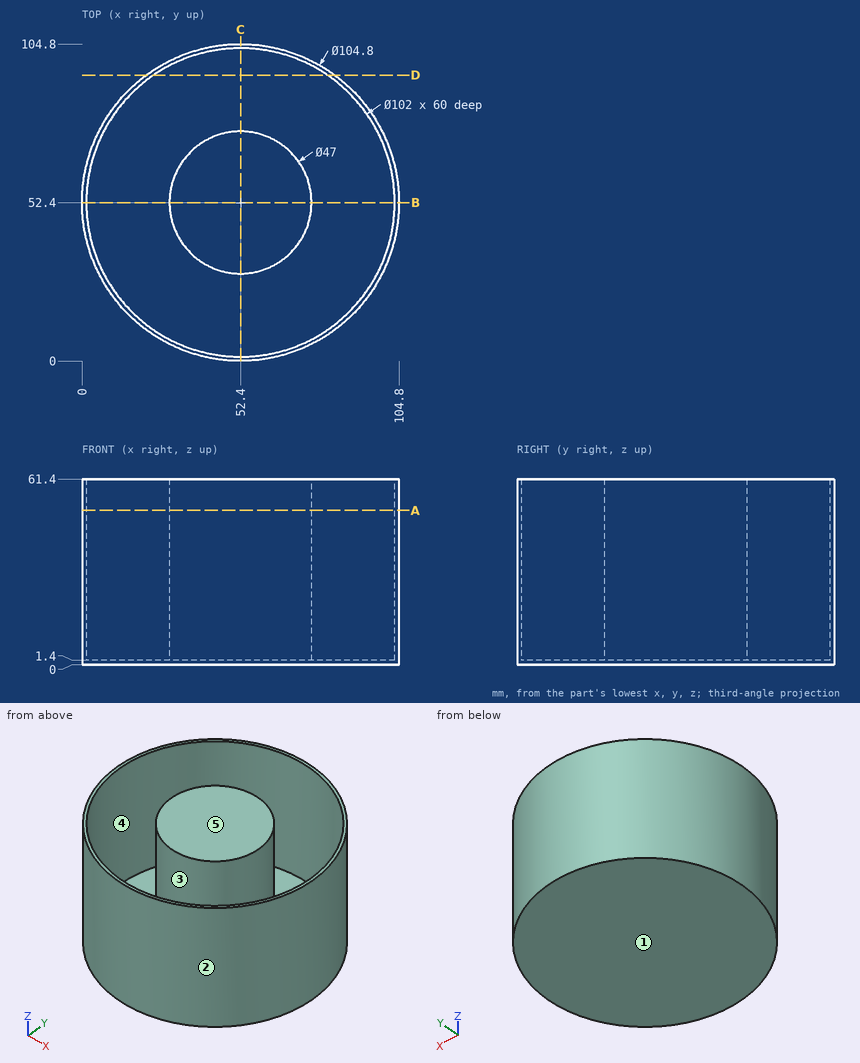
Can you work these out from the drawing? Everything is in mm from the part's minimum corner. A direction names the side the tool comes from. Give positions to 0.01 mm unless a question says otherwise; leave off trailing zeros. Order: outer loops, then holes, each group sorted by start corner. A loop starts at its lowest first (then second) coordinate and runs counter-clockwise, first axis right, second up. Notation, with made-up numbers: M -29.75,-2.5 L 25.25,-2.5 A12 cw 25.25,17.5 Z; hole C 67.5,30.25 d1. An arc over 180 degrees is marked long. One line per item, written item: value.
Item 1: Please list where these lines run through material, in increasing order: line 1 (Y direction, x = 52, z = 40); line 2 (X direction, y = 47.5, z = 53.5).
Verdict:
line 1: 0 to 1.4, 28.9 to 75.9, 103.4 to 104.8
line 2: 0.23 to 1.64, 29.42 to 75.38, 103.16 to 104.57
Item 2: If we section it at A-A on z = 51: Write out the boundary of the cut face in (x, y).
Verdict:
outline: C 52.4,52.4 d104.8; C 52.4,52.4 d47; hole C 52.4,52.4 d102
Item 3: For the marked faces 4 and 5, which set-ups out of +Z, -Z, +X, -X, +Y, -Y let a thin tool reach every point of the face, with its end or its side?
Verdict:
face 4: +Z
face 5: +Z, +X, -X, +Y, -Y
Item 4: If we section it at B-B on y = 52.4: Write out the boundary of the cut face in (x, z), and give its area (3 significant figures).
Verdict:
outline: M 0,0 L 104.8,0 L 104.8,61.4 L 103.4,61.4 L 103.4,1.4 L 75.9,1.4 L 75.9,61.4 L 28.9,61.4 L 28.9,1.4 L 1.4,1.4 L 1.4,61.4 L 0,61.4 Z
area: 3,130 mm2
Item 5: If we mould it in two halves opening along Y, with no side actions, what happens to the marked faces 1, 2 and 3? For each: pulls with the +Y half, pulls with the -Y half, needs draft (parallel to the pull), parting line crosses it, or undercut.
Verdict:
face 1: needs draft
face 2: parting line crosses it
face 3: undercut
Item 6: For pin 1 (2 mm diameter, centred on x = 33, z = 27, fed in from +Y); pin 2 (4 mm diameter, centred on x = 30.5, z = 21.5, fed in from +Y); pin 3 (6 mm diameter, centred on x = 25.5, z = 15.5, fed in from +Y), each with a flat end and sliding along its axis, tell me the tip position at first contact or that it passes through.
Verdict:
pin 1: y = 101.46
pin 2: y = 100.87
pin 3: y = 99.03
Item 7: If we section it at D-D on y = 94.5: Write out the boundary of the cut face in (x, z).
Verdict:
outline: M 21.2,0 L 83.6,0 L 83.6,61.4 L 81.19,61.4 L 81.19,1.4 L 23.61,1.4 L 23.61,61.4 L 21.2,61.4 Z
